Drawing for the job (mm, zero at the part's lowest x, y, z). Give positions to 0.01 mm unless a question says otherwise; leave off trailing zeros. Order: outer loops, then holes, each group sorted by start corner. A loop starts at its lowest first (then second) coordinate and runs counter-clockwise, first axis right, second up. Notation, with made-up numbers: (-27, 48.25) - (26, 48.25) arc R30 ccw to (26, 77.25) - close; hole circle Ø3 at (-6.5, 49). An arc over 180 degrees is marked (long way). Use a Markdown table: item, result. Add a question column.
(1) Wall check: line 1 (X direction, y = 9.75, z = 92.5); line 2 (X direction, y = 3.25, z = 89); line 3 (X direction, y = 7, z = 42.5). Give the ranges that are in metal, low to high.
(2) Flat gauge pins, fed straight in: pin 1 (3 mm diameter, centred on y = 2, z = 164.5, fed in from -X); pin 2 (1 mm diameter, centred on y = 4, z = 210, fed in from -X); pin 3 (5 mm diameter, centred on y = 7, z = 206, fed in from -X). Where does each tip first touch, or does it go through?
(3) Slice it at A-A (z = 251). Write the cut outline in (x, y).
(4) Slice it at B-B (y = 5). Write the cut outline in (x, z).
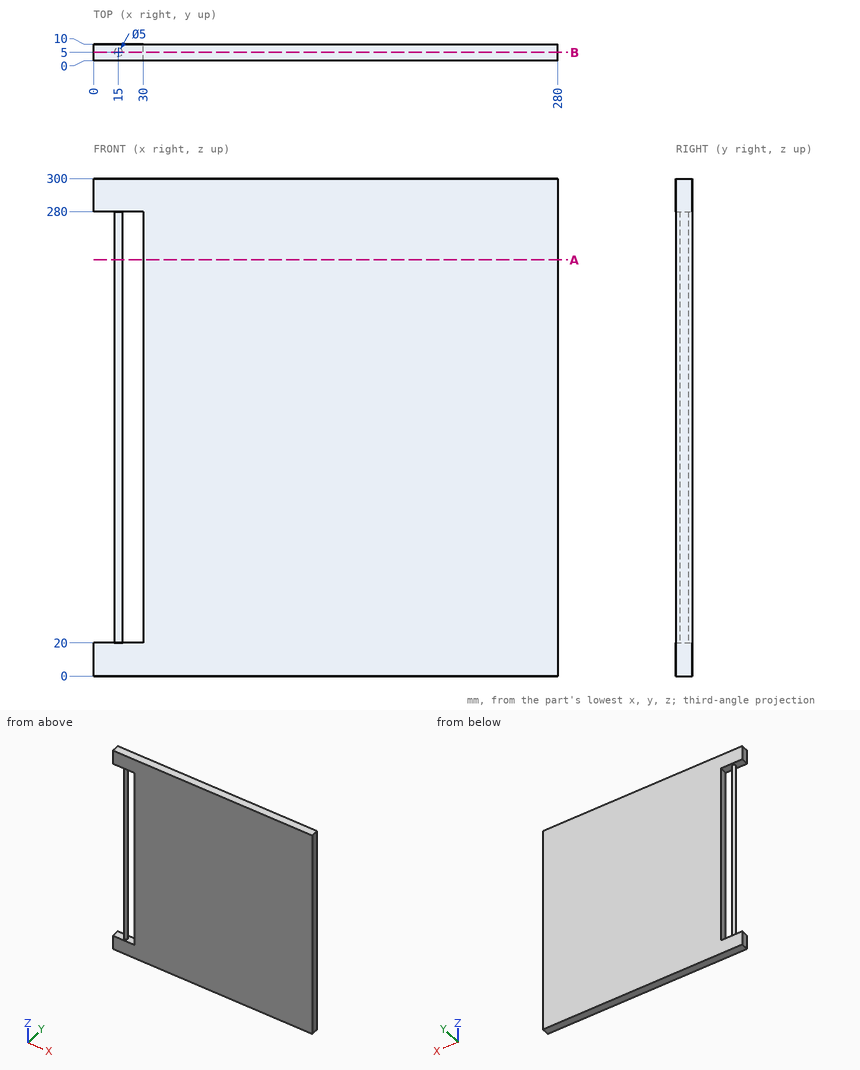
Solution:
| question | item | result |
|---|---|---|
| 1 | line 1 | 30 to 280 |
| 1 | line 2 | 13.21 to 16.79, 30 to 280 |
| 1 | line 3 | 13.5 to 16.5, 30 to 280 |
| 2 | pin 1 | x = 13 |
| 2 | pin 2 | x = 12.55 |
| 2 | pin 3 | x = 12.5 |
| 3 | outline | circle Ø5 at (15, 5); (30, 0) - (280, 0) - (280, 10) - (30, 10) - close |
| 4 | outline | (0, 0) - (280, 0) - (280, 300) - (0, 300) - (0, 280) - (12.5, 280) - (12.5, 20) - (0, 20) - close; hole (17.5, 20) - (30, 20) - (30, 280) - (17.5, 280) - close |
